The model under review builds one solid part; all positions refer to its coordinate system, in mm. A direction names the side the tool comes from. Coordinates: 2 decimals unless noted, no trailing zeros. Loops run counter-clockwise (first coordinate to the right, second up) from the corner with the lowest first, then second, coordinate; pieces in that order, holes last. Notation, with made-up numbers: M -6,27.5 L 5,27.5 A22 cw 5,64.5 Z; hole C -31,19.5 d3. An arc over 180 degrees is marked long. Use one line per item in the form item = value.
```python
from build123d import *

# Parameters (mm, degrees)
SKETCH2_W           = 90
SKETCH2_H           = 90
BOSS_EXTRUDE1_DEPTH = 20
SKETCH5_W           = 84.5
SKETCH5_H           = 84.5
CUT_EXTRUDE2_DEPTH  = 13
SKETCH13_W          = 84.5
SKETCH13_H          = 57
CUT_EXTRUDE5_DEPTH  = 6
SKETCH17_RX         = 10.196247106
SKETCH17_RY         = 2.793572888
CUT_EXTRUDE6_DEPTH  = 2.75
SKETCH25_W          = 84.5
SKETCH25_H          = 13.75
BOSS_EXTRUDE6_DEPTH = 14
SKETCH27_W          = 87.25
SKETCH27_H          = 87.25
SKETCH27_W_2        = 84.5
SKETCH27_H_2        = 84.5
BOSS_EXTRUDE8_DEPTH = 3


with BuildPart() as part:
    # Sketch2 → Boss-Extrude1 (new body)
    with BuildSketch(Plane(origin=(0, 0, 0), x_dir=(1, 0, 0), z_dir=(0, 1, 0))):
        Rectangle(SKETCH2_W, SKETCH2_H)
    extrude(amount=BOSS_EXTRUDE1_DEPTH)

    # Sketch5 → Cut-Extrude2 (cut)
    with BuildSketch(Plane(origin=(0, 20, 0), x_dir=(1, 0, 0), z_dir=(0, 1, 0))):
        Rectangle(SKETCH5_W, SKETCH5_H)
    extrude(amount=-CUT_EXTRUDE2_DEPTH, mode=Mode.SUBTRACT)

    # Sketch13 → Cut-Extrude5 (cut)
    with BuildSketch(Plane(origin=(0, 7, 0), x_dir=(1, 0, 0), z_dir=(0, 1, 0))):
        Rectangle(SKETCH13_W, SKETCH13_H)
    extrude(amount=-CUT_EXTRUDE5_DEPTH, mode=Mode.SUBTRACT)

    # Sketch17 → Cut-Extrude6 (cut)
    with BuildSketch(Plane(origin=(-45, -8.202038474, 0), x_dir=(0, 0, 1), z_dir=(-1, 0, 0))):
        with Locations(Location((0.657720021, 24.185537931), (0, 0, 180))):
            Ellipse(SKETCH17_RX, SKETCH17_RY)
    extrude(amount=-CUT_EXTRUDE6_DEPTH, mode=Mode.SUBTRACT)

    # Sketch25 → Boss-Extrude6 (add)
    with BuildSketch(Plane(origin=(0, 7, 0), x_dir=(1, 0, 0), z_dir=(0, 1, 0))):
        with Locations((0, 35.375)):
            Rectangle(SKETCH25_W, SKETCH25_H)
        with Locations((0, -35.375)):
            Rectangle(SKETCH25_W, SKETCH25_H)
    extrude(amount=BOSS_EXTRUDE6_DEPTH)

    # Sketch27 → Boss-Extrude8 (add)
    with BuildSketch(Plane(origin=(0, 20, 0), x_dir=(1, 0, 0), z_dir=(0, 1, 0))):
        Rectangle(SKETCH27_W, SKETCH27_H)
        Rectangle(SKETCH27_W_2, SKETCH27_H_2, mode=Mode.SUBTRACT)
    extrude(amount=BOSS_EXTRUDE8_DEPTH)


solid = part.part
```
1. Insertion check: P1, Ø1.5, axis at y = 21.5, z = 21.5, coming from the -X side (3 decimals); P2, Ø7, axis at x = -12, z = 37, coming from the +Y side; P3, Ø0.6, axis at x = -17, y = 22, coming from the -Z side (3 decimals); P4, Ø5, axis at x = -8.5, z = -5, coming from the -Y side. Each pin has a flat end and moves straight along its axis. Give the tip position at first contact, or say it passes through.
Response values:
P1 = -43.625
P2 = 21
P3 = -43.625
P4 = 0
2. Add section A-A (y = 8.5). State the section outline as (x, z) points.
Response values:
outline = M -45,-45 L 45,-45 L 45,45 L -45,45 Z; hole M -42.25,-28.5 L 42.25,-28.5 L 42.25,28.5 L -42.25,28.5 Z
3. The part is to be moulded in two halves that separate along Y. For faces 6 (the face through (-1, 10, -45)), 7 (the face through (-1, 1, 0)), 8 (the face through (-1, 0, -1)), say which applies: pulls with the +Y half, pulls with the -Y half, needs draft (parallel to the pull), parting line crosses it, or undercut.
Response values:
face_6 = needs draft
face_7 = pulls with the +Y half
face_8 = pulls with the -Y half
4. Wall thickness on line 1 along X through (y, z) = (7, 23.5); line 2 along Z through (x, y) = (4, 4.75); line 3 along Y through (x, z) = (-4.5, -21.5): over which ranges is each line inside the solid? List them lowest first. Write a range as from..to.
Response values:
line_1 = -45..-42.25, 42.25..45
line_2 = -45..-28.5, 28.5..45
line_3 = 0..1
5. Add section B-B (x = -5). State the section outline as (y, z) points (3 decimals).
Response values:
outline = M 0,-45 L 20,-45 L 20,-43.625 L 23,-43.625 L 23,-42.25 L 21,-42.25 L 21,-28.5 L 1,-28.5 L 1,28.5 L 21,28.5 L 21,42.25 L 23,42.25 L 23,43.625 L 20,43.625 L 20,45 L 0,45 Z
6. Add section C-C (z = 27). State the section outline as (x, y) points (3 decimals), then the cut area to 3 significant figures.
Response values:
outline = M -45,0 L 45,0 L 45,20 L 43.625,20 L 43.625,23 L 42.25,23 L 42.25,1 L -42.25,1 L -42.25,23 L -43.625,23 L -43.625,20 L -45,20 Z
area = 203 mm^2
7. Machinability: for faces 1 (the face through (-43.625, 21, 1)), 2 (the face through (-1, 21, 35)), 3 (the face through (-1, 21, -43.625)), 4 (the face through (-1, 21, 43.625)), 5 (the face through (-1, 10, 45)), which of the approach directions +Z, -Z, +X, -X, +Y, -Y give a long, thin tool a straight path to every point of the face, cutting with its end or side? Answer none if there is none.
Response values:
face_1 = +Z, -Z, -X, +Y
face_2 = +Y
face_3 = -Z, +X, -X, +Y
face_4 = +Z, +X, -X, +Y
face_5 = +Z, +X, -X, +Y, -Y
